Verification items for the finished model (mm, model axes). A direction names the side the tool comes from. Round coordinates to 2 decimals unless told otherwise and drop trailing zeros. Write each loop counter-clockwise with the first axis right and the second up, starting at its lowest first coordinate (ties: lowest second). Pieces come first, ordered by that corner, then holes. Notation, with made-up numbers: M -4,-27.5 L 12,-27.5 A28 ccw 12,6.5 Z; hole C 86.25,13.5 d11. An arc over 180 degrees is marked long. Answer in a Markdown table with one row per item. Add a question column.
1. Sectioned sample at B-B on z = 429. Record the cut outline in (x, y).
2. Go/stop test with flat-tipped pins: pin 1 Ø10 at (x, y) = (-17.83, 0) entering from +Z (3 decimals); pin 2 Ø10 at (y, z) = (48, 119.5) entering from -X; pin 3 Ø4 at (y, z) = (84, 195.5) entering from +X; pin 4 Ø4 at (y, z) = (133.5, 403) entering from -X. Record where each tip stops, or that it passes through.
3. Sectioned sample at C-C on x = 52. Record the cut outline in (y, z).
4. Draft check along X on faces 3 (the cylindrical face through (286.62, 304.726, 450.799)), 4 (the flat face through (289, 116, 12.7)), 5 (the flat face through (289, 121, 914.4)). Enter one of: pulls with the +X half, pulls with the -X half, needs draft (parallel to the pull), parting line crosses it, or undercut.
5. Sectioned sample at A-A on y = 96.5. Record the cut outline in (x, z), plus the area to 3 significant figures.
6. Set-up check for faces 1 (the flat face through (289, 116, 901.7)), 2 (the flat face through (289, 121, 0)): record each of +Z, -Z, +X, -X, +Y, -Y from which the full face is reachable in a straight line by a thin tool's end or side.
7. Material ranges on probe 1 along Z at (x, y) = (142, 97.5); probe 2 along X at (y, z) = (103, 602); probe 3 along X at (y, z) = (262, 535), recorded low to high.
8. Sectioned sample at D-D on y = 173. Record the cut outline in (x, z).
Autodesk Inventor part; units mm, degrees
ref_plane "YZ Plane" through (0, 0, 0) normal (1, 0, 0) x (0, 1, 0)
ref_plane "XZ Plane" through (0, 0, 0) normal (0, 1, 0) x (-1, 0, 0)
ref_plane "XY Plane" through (0, 0, 0) normal (0, 0, 1) x (1, 0, 0)
sketch "Sketch1" plane through (0, 0, 0) normal (0, 0, 1) x (1, 0, 0)
  arc A0 (598.1223, 0) -> (-11.4777, 0) centre (293.3223, 0) ccw
  line L0 (-11.4777, 0) -> (598.1223, 0)
  point P0 (0, 0)
  dimension "d0" = 609.6
  dimension "d1" = 304.8
extrude "Extrusion1" add sketch "Sketch1" along normal blind 914.4
shell "Shell1" thickness 12.7 removed faces 1 at (191.7223, 0, 609.6)
ref_plane "Work Plane1" through (0, 0, 812.8) normal (0, 0, 1) x (1, 0, 0)
ref_plane "Work Plane2" through (0, 0, 101.6) normal (0, 0, -1) x (-1, 0, 0)
sketch "Sketch2" plane through (0, 0, 101.6) normal (0, 0, -1) x (-1, 0, 0)
  circle A0 centre (17.8277, 0) radius 10.16
  circle A1 centre (17.8277, 0) radius 6.35
  arc A2 (11.4777, 0) -> (-598.1223, 0) centre (-293.3223, 0) ccw
  point P0 (0, 0)
  dimension "d7" = 20.32
  dimension "d8" = 12.7
extrude "Extrusion2" add sketch "Sketch2" against normal blind 50.8
sketch "Sketch3" plane through (0, 0, 812.8) normal (0, 0, 1) x (1, 0, 0)
  arc A0 (-11.3766, 7.8491) -> (-7.6677, 0) centre (-17.8277, 0) ccw
  circle A1 centre (-17.8277, 0) radius 10.16
  circle A2 centre (-17.8277, 0) radius 6.35
  point P0 (0, 0)
  point P1 (-7.6677, 0)
  dimension "d11" = 12.7
extrude "Extrusion3" add sketch "Sketch3" against normal blind 50.8
properties part number "chestTop"
Geometry check:
| question | item | result |
|---|---|---|
| 1 | outline | M -11.48,0 L 1.22,0 A292.1 cw 585.42,0 L 598.12,0 A304.8 ccw Z |
| 2 | pin 1 | passes through |
| 2 | pin 2 | stops at x = -8.43 |
| 2 | pin 3 | stops at x = 586.88 |
| 2 | pin 4 | stops at x = 18.35 |
| 3 | outline | M 0,0 L 186.19,0 L 186.19,914.4 L 0,914.4 L 0,901.7 L 164.58,901.7 L 164.58,12.7 L 0,12.7 Z |
| 4 | face 3 | parting line crosses it |
| 4 | face 4 | undercut |
| 4 | face 5 | needs draft |
| 5 | outline | M 4.2,0 L 582.44,0 L 582.44,914.4 L 4.2,914.4 Z; hole M 17.62,12.7 L 569.02,12.7 L 569.02,901.7 L 17.62,901.7 Z |
| 5 | area | 38,600 mm2 |
| 6 | face 1 | -Y |
| 6 | face 2 | -Z, +X, -X, +Y, -Y |
| 7 | probe 1 | z = 0 to 12.7, 901.7 to 914.4 |
| 7 | probe 2 | x = 6.45 to 19.98, 566.66 to 580.19 |
| 7 | probe 3 | x = 137.57 to 164.18, 422.47 to 449.08 |
| 8 | outline | M 42.38,0 L 544.27,0 L 544.27,914.4 L 42.38,914.4 Z; hole M 57.96,12.7 L 528.68,12.7 L 528.68,901.7 L 57.96,901.7 Z |
